```python
from build123d import *

# Parameters (mm, degrees)
SKETCH1_R           = 1.25
BOSS_EXTRUDE1_DEPTH = 13.86
SKETCH1_3_R         = 3.44
BOSS_EXTRUDE2_DEPTH = 2.5
SKETCH1_4_R         = 2.74
BOSS_EXTRUDE3_DEPTH = 3.5
SKETCH1_5_R         = 1
BOSS_EXTRUDE4_DEPTH = 14.75


with BuildPart() as part:
    # Sketch1 → Boss-Extrude1 (new body)
    with BuildSketch(Plane.XY):
        with BuildLine():
            Line((-9, 11.15), (9, 11.15))
            ThreePointArc((9, 11.15), (10.767766953, 10.417766953), (11.5, 8.65))
            Line((11.5, 8.65), (11.5, -28.35))
            ThreePointArc((11.5, -28.35), (10.767766953, -30.117766953), (9, -30.85))
            Line((9, -30.85), (-9, -30.85))
            ThreePointArc((-9, -30.85), (-10.767766953, -30.117766953), (-11.5, -28.35))
            Line((-11.5, -28.35), (-11.5, 8.65))
            ThreePointArc((-11.5, 8.65), (-10.767766953, 10.417766953), (-9, 11.15))
        make_face()
        with Locations((-9, 8.65)):
            Circle(SKETCH1_R, mode=Mode.SUBTRACT)
        with Locations((9, 8.65)):
            Circle(SKETCH1_R, mode=Mode.SUBTRACT)
    extrude(amount=-BOSS_EXTRUDE1_DEPTH)

    # Sketch1_3 → Boss-Extrude2 (add)
    with BuildSketch(Plane.XY):
        Circle(SKETCH1_3_R)
    extrude(amount=BOSS_EXTRUDE2_DEPTH)

    # Sketch1_4 → Boss-Extrude3 (add)
    with BuildSketch(Plane.XY):
        Circle(SKETCH1_4_R)
    extrude(amount=BOSS_EXTRUDE3_DEPTH)

    # Sketch1_5 → Boss-Extrude4 (add)
    with BuildSketch(Plane.XY):
        with BuildLine():
            ThreePointArc((2.74, 0), (2.556417641, 0.986067362), (2.030270918, 1.84))
            Line((2.030270918, 1.84), (-2.030270918, 1.84))
            ThreePointArc((-2.030270918, 1.84), (-2.74, 0), (-2.030270918, -1.84))
            Line((-2.030270918, -1.84), (2.030270918, -1.84))
            ThreePointArc((2.030270918, -1.84), (2.556417641, -0.986067362), (2.74, 0))
        make_face()
        Circle(SKETCH1_5_R, mode=Mode.SUBTRACT)
    extrude(amount=BOSS_EXTRUDE4_DEPTH)


solid = part.part
```
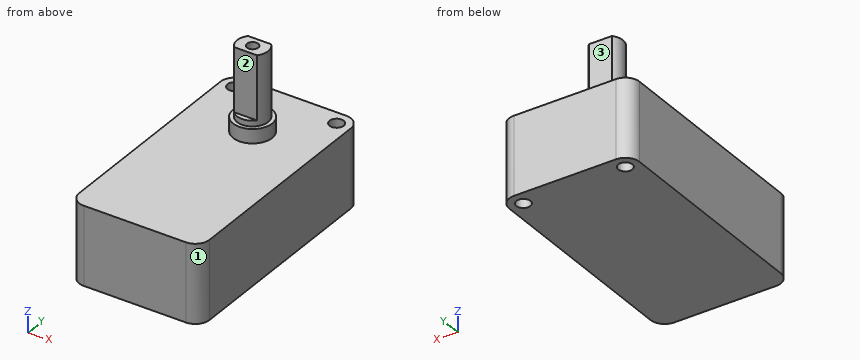
The model under review builds one solid part; all positions refer to its coordinate system, in mm. Face numbers are marked on the shaded views. A direction names the side the tool comes from. Round coordinates to 2 decimals unless told otherwise and drop trailing zeros. Loops run counter-clockwise (first coordinate to the right, second up) from the corner with the lowest first, then second, coordinate; pieces in that order, holes last. Notation, with made-up numbers: (36.25, 27) -> (48.25, 27) arc R13 cw to (48.25, 38) -> close; hole circle Ø5 at (18.5, -8). An arc over 180 degrees is marked (long way). Answer as a JSON object with one key per item and string values. Group by question number.
1) For pin 1 Ø1 at (x, y) = (0, 0) entering from +Z; pin 2 Ø4.5 at (x, z) = (-0.5, 9) entering from +Y; pin 3 Ø1.2 at (x, z) = (0.5, 8.5) entering from -Y, all flat-tipped, find the tip position at first contact; note any pin that passes through.
2) For line 1 (Y direction, x = 0, z = 11); line 2 (X direction, y = 0, z = 7); line 3 (Z direction, x = -9, y = -27), list the stretches that pass through material, from the lowest coordinate up. Write a range as [from, to].
3) We need section C-C on x = -7.25. Write out the cut boundary in (y, z).
4) We need section A-A on z = -11.5. Write out the cut boundary in (x, y).
5) We need section D-D on y = -18. Write out the cut boundary in (x, z), then the cut area to 3 significant figures.
6) For the marked faces 1, 2 and 3, list the 3-axis set-ups (+Z, -Z, +X, -X, +Y, -Y) from which the entire face can be reached by the end or side of a thin tool; tool diameter is ignored.
7) We need section B-B on z = 4.25. Write out the cut boundary in (x, y).
Result set:
{
 "1": {"pin 1": "z = 3.5", "pin 2": "y = 1.84", "pin 3": "y = -1.84"},
 "2": {"line 1": "[-1.84, -1], [1, 1.84]", "line 2": "[-2.74, -1], [1, 2.74]", "line 3": "[-13.86, 0]"},
 "3": {"outline": "(-30.85, -13.86) -> (11.15, -13.86) -> (11.15, 0) -> (-30.85, 0) -> close"},
 "4": {"outline": "(-11.5, -28.35) arc R2.5 ccw to (-9, -30.85) -> (9, -30.85) arc R2.5 ccw to (11.5, -28.35) -> (11.5, 8.65) arc R2.5 ccw to (9, 11.15) -> (-9, 11.15) arc R2.5 ccw to (-11.5, 8.65) -> close; hole circle Ø2.5 at (-9, 8.65); hole circle Ø2.5 at (9, 8.65)"},
 "5": {"outline": "(-11.5, -13.86) -> (11.5, -13.86) -> (11.5, 0) -> (-11.5, 0) -> close", "area": "319 mm²"},
 "6": {"face 1": "+Z, -Z, +X, -Y", "face 2": "+Z, +X, -X, -Y", "face 3": "+Z, +X, -X, +Y"},
 "7": {"outline": "(-2.03, -1.84) -> (2.03, -1.84) arc R2.74 ccw to (2.03, 1.84) -> (-2.03, 1.84) arc R2.74 ccw to start; hole circle Ø2 at (0, 0)"}
}
